Source: CAD feature listing. Evaluate the final solid. Frame: model axes, mm. A direction names the side the tool comes from. Round coordinates to 2 decimals unless told otherwise and drop trailing zeros. Write each loop counter-clockwise with the first axis right and the second up, starting at its lowest first coordinate (ties: lowest second). Pieces come first, ordered by that corner, then holes. Notation, with made-up numbers: (-34, 71) -> (10, 71) arc R10 cw to (10, 82) -> close; hole circle Ø7 at (-12.75, -11.75). An arc over 180 degrees is marked (long way). Return JSON: item names as keys, results as strings. Group by question number.
from build123d import *

# Parameters (mm, degrees)
F1_DEPTH  = 100
F2_W      = 30.510824
F2_H      = 31.205505
F3_DEPTH  = 25
F5_DEPTH  = 156.006396
F6_DEPTH  = 156.006396
F7_W      = 37.313528
F7_H      = 100
F7_H_2    = 62.66261
F8_DEPTH  = 15
F9_R      = 4.65702
F10_DEPTH = 25
F11_R     = 3.230766
F12_DEPTH = 130


with BuildPart() as f1:
    # F0 (on Top) → F1 (new body)
    with BuildSketch(Plane.XY):
        Polygon((56.264594, -78.003198), (88.659361, -78.003198), (88.659361, 78.003198), (-88.659361, 78.003198), (-88.659361, -78.003198), (30.689791, -78.003198), (30.689791, -63.084543), (-72.03573, -63.084543), (-72.03573, 63.084543), (72.03573, 63.084543), (72.03573, -63.084543), (56.264594, -63.084543), align=None)
    extrude(amount=F1_DEPTH)

    # F2 (on face) → F3 (cut)
    with BuildSketch(Plane.XZ.offset(78.003198)):
        with Locations((-28.984785, 51.321357)):
            Rectangle(F2_W, F2_H)
    extrude(amount=-F3_DEPTH, mode=Mode.SUBTRACT)

    # F4 (on face) → F5 (join, through all)
    with BuildSketch(Plane.XZ.offset(78.003198)):
        Polygon((88.659361, 100), (0, 155.675024), (-88.659361, 100), (30.689791, 100), (56.264594, 100), align=None)
    extrude(amount=-F5_DEPTH)

    # F4 (on face) → F6 (join, through all)
    with BuildSketch(Plane.XZ.offset(78.003198)):
        Polygon((-88.659361, 100), (0, 155.675024), (88.659361, 100), (91.31838, 104.234338), (0, 161.579134), (-91.31838, 104.234338), align=None)
    extrude(amount=-F6_DEPTH)

    # F7 (on face) → F8 (join)
    with BuildSketch(Plane.YZ.offset(88.659361)):
        with Locations((-18.656764, 50)):
            Rectangle(F7_W, F7_H)
        with Locations((-18.656764, 131.331305)):
            Rectangle(F7_W, F7_H_2)
    extrude(amount=F8_DEPTH)

    # F9 (on face) → F10 (join)
    with BuildSketch(Plane.XY.offset(162.66261)):
        with Locations((96.159361, -18.656764)):
            Circle(F9_R)
    extrude(amount=F10_DEPTH)

    # F11 (on face) → F12 (cut)
    with BuildSketch(Plane.XY.offset(187.66261)):
        with Locations((96.159361, -18.656764)):
            Circle(F11_R)
    extrude(amount=-F12_DEPTH, mode=Mode.SUBTRACT)


solid = f1.part
Item 1: Cut plane D-D on z = 14. Output: boundary loops of the cut face in (x, y).
Item 2: Cut plane A-A on z = 60.5. Output: boundary loops of the cut face in (x, y), and give its area (3 significant figures).
Item 3: First-contact query: pin 1 Ø11 at (y, z) = (-23, 134) entering from -X; pin 2 Ø16.5 at (x, y) = (-24.5, -69.5) entering from +Z; pin 3 Ø6 at (y, z) = (-62.5, 115) entering from -X. Flat tips, straight axial feed; report the tip coordinate or a pass-through.
Item 4: Cut plane C-C on x = -21.5. Output: boundary loops of the cut face in (y, z).
Item 5: Pull-direction query (X, two-part tool) for faces 1 (the flat face through (103.659, -19, 82)), 2 (the flat face through (95, -22, 187.663)), 3 (the flat face through (-88.659, 1, 49)), 4 (the flat face through (72.036, 1, 49)); classes: +X half, -X half, draft (parallel to the pull), parting line (faces both ways), or undercut.
Item 6: Set-up query: faces 5 (the flat face through (56.265, -70, 49)), 6 (the cylindrical face through (99.144, -19.894, 123.573)), 7 (the flat face through (64, -63.085, 49)). Return all of +Z, -Z, +X, -X, +Y, -Y with unobstructed straight access to the full face (end or side cutting, diameter ignored); none if empty.
Item 7: Cut plane B-B on y = 48.5. Output: boundary loops of the cut face in (x, z).
Item 8: Material intervals for probe 1 along X at (y, z) = (-55.5, 96); probe 2 along Y at (x, z) = (26.5, 68.5); probe 3 along X at (y, z) = (-26, 24), sorted ascending.
Here are the results:
{
 "1": {"outline": "(-88.66, -78) -> (30.69, -78) -> (30.69, -63.08) -> (-72.04, -63.08) -> (-72.04, 63.08) -> (72.04, 63.08) -> (72.04, -63.08) -> (56.26, -63.08) -> (56.26, -78) -> (88.66, -78) -> (88.66, -37.31) -> (103.66, -37.31) -> (103.66, 0) -> (88.66, 0) -> (88.66, 78) -> (-88.66, 78) -> close"},
 "2": {"outline": "(-88.66, -78) -> (-44.24, -78) -> (-44.24, -63.08) -> (-72.04, -63.08) -> (-72.04, 63.08) -> (72.04, 63.08) -> (72.04, -63.08) -> (56.26, -63.08) -> (56.26, -78) -> (88.66, -78) -> (88.66, -37.31) -> (103.66, -37.31) -> (103.66, 0) -> (88.66, 0) -> (88.66, 78) -> (-88.66, 78) -> close; (-13.73, -78) -> (30.69, -78) -> (30.69, -63.08) -> (-13.73, -63.08) -> close; hole circle Ø6.46 at (96.16, -18.66)", "area": "9,180 mm^2"},
 "3": {"pin 1": "stops at x = -52.68", "pin 2": "stops at z = 151.37", "pin 3": "stops at x = -78.95"},
 "4": {"outline": "(-78, 0) -> (-63.08, 0) -> (-63.08, 35.72) -> (-78, 35.72) -> close; (-78, 66.92) -> (-63.08, 66.92) -> (-63.08, 100) -> (63.08, 100) -> (63.08, 0) -> (78, 0) -> (78, 148.08) -> (-78, 148.08) -> close"},
 "5": {"face 1": "+X half", "face 2": "draft", "face 3": "-X half", "face 4": "undercut"},
 "6": {"face 5": "-Z, -Y", "face 6": "+Z", "face 7": "-Z"},
 "7": {"outline": "(-91.32, 104.23) -> (-88.66, 100) -> (-88.66, 0) -> (-72.04, 0) -> (-72.04, 100) -> (72.04, 100) -> (72.04, 0) -> (88.66, 0) -> (88.66, 100) -> (91.32, 104.23) -> (0, 161.58) -> close"},
 "8": {"probe 1": "x = -88.66 to -72.04, 72.04 to 88.66", "probe 2": "y = -78 to -63.08, 63.08 to 78", "probe 3": "x = -88.66 to -72.04, 72.04 to 103.66"}
}
